from build123d import *

# Parameters (mm, degrees)
BOSS_EXTRUDE3_DEPTH     = 31
SKETCH2_R               = 12.7
CUT_EXTRUDE1_DEPTH      = 317.5
CUT_EXTRUDE3_DEPTH      = 416.807816184
CUT_EXTRUDE3_DEPTH_BACK = 416.807816184
SKETCH6_R               = 12.7
SKETCH3_R               = 19.05
CUT_EXTRUDE4_DEPTH      = 15.24
SKETCH7_R               = 5
CUT_EXTRUDE5_DEPTH      = 25.4


with BuildPart() as part:
    # Sketch5 → Boss-Extrude3 (new, symmetric)
    with BuildSketch(Plane.XY):
        Polygon((76.2, 266.7), (-317.5, 266.7), (-317.5, -190.5), (-114.3, -190.5), (-114.3, 25.4), (-50.8, 25.4), (-50.8, -25.4), (50.8, -25.4), (50.8, 25.4), (76.2, 25.4), align=None)
    extrude(amount=BOSS_EXTRUDE3_DEPTH, both=True)

    # Sketch2 → Cut-Extrude1 (cut)
    with BuildSketch(Plane(origin=(-317.5, 0, -457.2), x_dir=(0, 0, -1), z_dir=(1, 0, 0))):
        with Locations(Location((-457.2, 0, 0), (0, 0, 90))):
            Circle(SKETCH2_R)
    extrude(amount=CUT_EXTRUDE1_DEPTH, mode=Mode.SUBTRACT)

    # Sketch6 → Cut-Extrude3 (cut, two sides: drawn at the far end of the back side and taken through both)
    with BuildSketch(Plane(origin=(0, 0, 0), x_dir=(1, 0, 0), z_dir=(0, 1, 0)).offset(-CUT_EXTRUDE3_DEPTH_BACK)):
        with Locations(Location((0, 0, 0), (0, 0, 270))):
            Circle(SKETCH6_R)
    extrude(amount=CUT_EXTRUDE3_DEPTH + CUT_EXTRUDE3_DEPTH_BACK, mode=Mode.SUBTRACT)

    # Sketch3 → Cut-Extrude4 (cut)
    with BuildSketch(Plane(origin=(-317.5, 0, -457.2), x_dir=(0, 0, -1), z_dir=(1, 0, 0))):
        with Locations(Location((-457.2, 0, 0), (0, 0, 180))):
            Circle(SKETCH3_R)
    extrude(amount=CUT_EXTRUDE4_DEPTH, mode=Mode.SUBTRACT)

    # Sketch7 → Cut-Extrude5 (cut)
    with BuildSketch(Plane.XZ.offset(190.5)):
        with Locations((-291.304206057, 21.825)):
            Circle(SKETCH7_R)
        with Locations((-291.304206057, -21.825)):
            Circle(SKETCH7_R)
        with Locations((-241.304206057, 21.825)):
            Circle(SKETCH7_R)
        with Locations((-241.304206057, -21.825)):
            Circle(SKETCH7_R)
        with Locations((-191.304206057, 21.825)):
            Circle(SKETCH7_R)
        with Locations((-191.304206057, -21.825)):
            Circle(SKETCH7_R)
    extrude(amount=-CUT_EXTRUDE5_DEPTH, mode=Mode.SUBTRACT)


solid = part.part
Can you work these out from the model? Positions are in its coordinate system, mm. A direction names the side the tool comes from. Give positions to 0.01 mm unless a question says otherwise; leave off trailing zeros. Loops run counter-clockwise (first coordinate to the right, second up) from the corner with the lowest first, then second, coordinate; pieces in that order, holes last. Notation, with made-up numbers: M 30,47.25 L 76,47.25 A20 cw 76,63.25 Z; hole C 20.25,77.25 d5. An arc over 180 degrees is marked long. One line per item, written item: value.
1) Imagine slicing it at A-A on y = 0. Write out the boundary of the cut face in (x, z), and give its area (3 significant figures).
Geometry check:
outline: M -317.5,-31 L -114.3,-31 L -114.3,-12.7 L -302.26,-12.7 L -302.26,-19.05 L -317.5,-19.05 Z; M -317.5,19.05 L -302.26,19.05 L -302.26,12.7 L -114.3,12.7 L -114.3,31 L -317.5,31 Z; M -50.8,-31 L 50.8,-31 L 50.8,31 L -50.8,31 L -50.8,12.7 L 0,12.7 A12.7 cw 0,-12.7 L -50.8,-12.7 Z
area: 12,000 mm²
2) Please list where these lines run through material, in increasing order: line 1 (X direction, y = 154, z = 0); line 2 (Y direction, x = -37.5, z = 0); line 3 (Z direction, x = 0, y = 173.5).
Geometry check:
line 1: x = -317.5 to -12.7, 12.7 to 76.2
line 2: y = -25.4 to -12.7, 12.7 to 266.7
line 3: z = -31 to -12.7, 12.7 to 31
3) Thinking about a two-plate mould opening in Y: for faces 1 (the face through (-191, -165.1, 22)), 2 (the face through (-50.8, 12, 7)), 3 (the face through (-302.26, 12.4, 4)), which applies, +Y half, -Y half, draft (parallel to the pull), parting line (faces both ways), or undercut?
Geometry check:
face 1: -Y half
face 2: draft
face 3: undercut
4) Imagine slicing it at C-C on y = 172.5. Write out the boundary of the cut face in (x, z), and give its area (3 significant figures).
Geometry check:
outline: M -317.5,-31 L 76.2,-31 L 76.2,31 L -317.5,31 Z; hole C 0,0 d25.4
area: 23,900 mm²
5) On a 3-axis mill with a long thin cutter (end or side, diameter ignored), from which of +Z, -Z, +X, -X, +Y, -Y can I reach the whole of each face in a straight line? I mean faces 4 (the face through (63, 25.4, 0)), 5 (the face through (-236.535, -177.978, 23.327)), 6 (the face through (-118, 266.7, 0)), 7 (the face through (-209.6, -10.1, -7.7)). Say none if no direction works.
Geometry check:
face 4: +Z, -Z, +X, -Y
face 5: -Y
face 6: +Z, -Z, +X, -X, +Y
face 7: -X
6) I'm going to push flat-ended pins straight in: pin 1 (5 mm diameter, centred on x = -243, z = 22, fed in from -Y); pin 2 (20.5 mm diameter, centred on x = 59, z = -11, fed in from -Y); pin 3 (11.5 mm diameter, centred on x = -191.3, z = 21.82, fed in from -Y); pin 4 (1 mm diameter, centred on y = -106, z = -6, fed in from +X). Where does each tip first touch, or does it pass through?
Geometry check:
pin 1: stops at y = -165.1
pin 2: stops at y = -25.4
pin 3: stops at y = -190.5
pin 4: stops at x = -114.3
7) Imagine slicing it at B-B on x = -25. Write out the boundary of the cut face in (y, z).
Geometry check:
outline: M -25.4,-31 L 266.7,-31 L 266.7,31 L -25.4,31 Z; hole C 0,0 d25.4
8) Imagine slicing it at D-D on x = -70.5. Write out the boundary of the cut face in (y, z).
Geometry check:
outline: M 25.4,-31 L 266.7,-31 L 266.7,31 L 25.4,31 Z
